Input: part model. Units: mm. Frame: model coordinates. Face numbers are marked on the shaded views. A direction names the side the tool comes from. Give positions to 0.01 mm unless a question says otherwise; leave off trailing zeros. Loops run counter-clockwise (first coordinate to the right, second up) from the corner with the lowest first, then second, coordinate; pieces in that order, holes last. Notation, with made-up numbers: (-9, 65.5) -> (4, 65.5) arc R10 cw to (4, 72.5) -> close; hole circle Ø7 at (-35.5, -29.75). An arc over 180 degrees is marked (long way). Use CSV: the item, a comma, the result in double quotes.
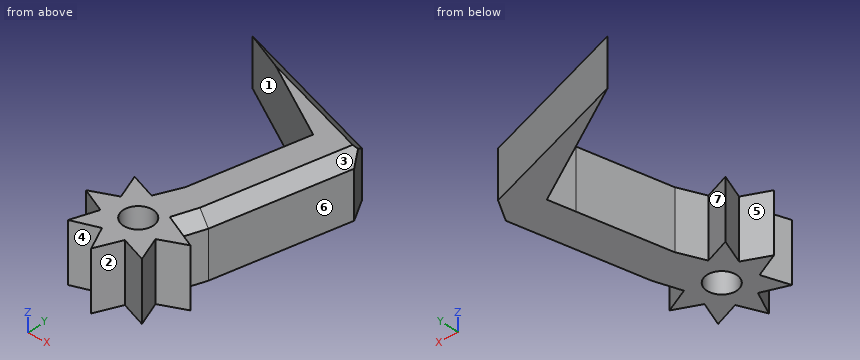
Autodesk Fusion 360 part; units mm, degrees
sketch "Sketch1" plane through (0, 0, 0) normal (0, 0, 1) x (1, 0, 0)
  line L0 (29.7102, -20.9929) -> (0, -20.9929)
  line L1 (-7, 31.5) -> (20.239, 31.5)
  line L2 (20.239, 31.5) -> (29.7102, -20.9929)
  line L3 (-7, 31.5) -> (0, -20.9929)
  line L4 (3.9378, -2.5628) -> (1.375, -8.75)
  line L5 (1.375, -8.75) -> (3.9378, -14.9372)
  line L6 (3.9378, -14.9372) -> (10.125, -17.5)
  line L7 (10.125, -17.5) -> (16.3122, -14.9372)
  line L8 (16.3122, -14.9372) -> (18.875, -8.75)
  line L9 (18.875, -8.75) -> (16.3122, -2.5628)
  line L10 (16.3122, -2.5628) -> (10.125, 0)
  line L11 (15.1989, 4.3652) -> (15.1875, 4.3554)
  line L12 (-7, 31.5) -> (14.4889, 18.96)
  line L13 (-7, 31.5) -> (21.9586, 21.9692)
  line L14 (21.9586, 21.9692) -> (16.3122, -2.5628)
  line L15 (10.125, 0) -> (13.5018, 14.6711)
  line L16 (10.125, 0) -> (3.9378, -2.5628)
  circle A0 centre (10.125, -8.75) radius 2.5
  circle A1 centre (10.125, -8.75) radius 5
  line L17 (7.0314, -1.2814) -> (10.125, -8.75) construction
  line L18 (10.125, 0) -> (8.2116, -4.1306)
  line L19 (8.2116, -4.1306) -> (3.9378, -2.5628)
  line L20 (3.9378, -2.5628) -> (5.5056, -6.8366)
  line L21 (5.5056, -6.8366) -> (1.375, -8.75)
  line L22 (1.375, -8.75) -> (5.5056, -10.6634)
  line L23 (5.5056, -10.6634) -> (3.9378, -14.9372)
  line L24 (3.9378, -14.9372) -> (8.2116, -13.3694)
  line L25 (8.2116, -13.3694) -> (10.125, -17.5)
  line L26 (10.125, -17.5) -> (12.0384, -13.3694)
  line L27 (12.0384, -13.3694) -> (16.3122, -14.9372)
  line L28 (16.3122, -14.9372) -> (14.7444, -10.6634)
  line L29 (14.7444, -10.6634) -> (18.875, -8.75)
  line L30 (18.875, -8.75) -> (14.7444, -6.8366)
  line L31 (14.7444, -6.8366) -> (16.3122, -2.5628)
  line L32 (16.3122, -2.5628) -> (12.0384, -4.1306)
  line L33 (12.0384, -4.1306) -> (10.125, 0)
  line L34 (13.5018, 14.6711) -> (14.4889, 18.96)
  point P0 (10.125, -8.75)
  dimension "d3" = 5
  dimension "d4" = 10
  dimension "d6" = 360
extrude "Extrude1" add sketch "Sketch1" along normal blind 10 contours L10 L12 L13 L14 L15 L34 | L10 L32 L33 | A1 L31 L32 | A1 L29 L30 | A1 L18 L33 | A1 | A1 L27 L28 | A1 L19 L20 | A1 L25 L26 | A1 L21 L22 | A1 L23 L24
chamfer "Chamfer1" distance 3 angle 45 1 edges at (21.9586, 21.9692, 5)
chamfer "Chamfer2" distance 2 angle 45 1 edges at (6.0545, 27.2035, 10)
chamfer "Chamfer3" distance 2 angle 45 2 edges at (15.5283, -4.6997, 10) (18.7989, 8.2414, 10)
1) Section query C-C (y = 17.5). Return loops of the section in (x, z), then the cut area to 3 significant figures.
From the geometry:
outline,"(14.15, 0) -> (20.93, 0) -> (20.93, 8) -> (18.88, 10) -> (14.15, 10) -> close"
area,"65.7 mm^2"
2) Section query A-A (z = 4.75). Return loops of the section in (x, y) (3 decimals), then the cut area to 3 significant figures.
From the geometry:
outline,"(-7, 31.5) -> (14.489, 18.96) -> (13.502, 14.671) -> (10.125, 0) -> (8.212, -4.131) -> (3.938, -2.563) -> (5.506, -6.837) -> (1.375, -8.75) -> (5.506, -10.663) -> (3.938, -14.937) -> (8.212, -13.369) -> (10.125, -17.5) -> (12.038, -13.369) -> (16.312, -14.937) -> (14.744, -10.663) -> (18.875, -8.75) -> (14.744, -6.837) -> (16.312, -2.563) -> (21.286, 19.046) -> (19.109, 22.907) -> close; hole circle Ø5 at (10.125, -8.75)"
area,"347 mm^2"
3) Section query B-B (x = 11.25). Return loops of the section in (y, z).
From the geometry:
outline,"(-15.07, 0) -> (-10.98, 0) -> (-10.98, 10) -> (-15.07, 10) -> close; (-6.52, 0) -> (4.89, 0) -> (4.89, 10) -> (-6.52, 10) -> close; (20.85, 0) -> (25.49, 0) -> (25.49, 8) -> (23.39, 10) -> (20.85, 10) -> close"
4) Reachability of the marked faces 4, 5, 6 and 7 from +Z, -Z, +X, -X, +Y, -Y: full face, straight path, thin tool, end or side. Return the list, or none.
From the geometry:
face 4,"+Z, -Z, -Y"
face 5,"+Z, -Z, -X"
face 6,"+Z, -Z, +X"
face 7,"+Z, -Z"
5) Section query D-D (x = -0.25). Return loops of the section in (y, z).
From the geometry:
outline,"(27.56, 0) -> (29.28, 0) -> (29.28, 8) -> (27.56, 9.63) -> close"
6) Mould query, pull axis X, two halves, no side actions, for the marked faces 1, 2 and 3. Classes: pulls with the +X half, pulls with the -X half, needs draft (parallel to the pull), parting line crosses it, or undercut.
From the geometry:
face 1,"pulls with the -X half"
face 2,"undercut"
face 3,"pulls with the +X half"
7) Ray query, line 1 (Y direction, x = 8, z = 2.5); line 2 (Y direction, x = 3, z = 3.75); line 3 (X direction, y = -7.5, z = 6). Return the intervals inside material, ascending.
From the geometry:
line 1,"y = -13.45 to -10.07, -7.43 to -4.05, 22.75 to 26.56"
line 2,"y = -9.5 to -8, 25.66 to 28.21"
line 3,"x = 4.07 to 7.96, 12.29 to 16.18"
8) Contact query for flat-ended pins moving along their axis: pin 1 (6 mm diameter, centred on x = 5.5, y = 20.5, fed in from +Z); pin 2 (2 mm diameter, centred on y = 1.5, z = 4.5, fed in from +X); pin 3 (6 mm diameter, centred on y = 12.5, z = 5, fed in from -X); pin 4 (1.5 mm diameter, centred on x = -3.5, z = 7, fed in from +Y). Output: stop coordinate, or through.
From the geometry:
pin 1,"passes through"
pin 2,"stops at x = 17.48"
pin 3,"stops at x = 12.31"
pin 4,"stops at y = 30.59"
